Read the model definition and answer for the solid it produces. Units are mm, in the model's axes. A direction names the side the tool comes from. Coordinates: 2 decimals unless noted, no trailing zeros. Order: outer loops, then holes, each group sorted by start corner. A loop starts at its lowest first (then second) coordinate and runs counter-clockwise, first axis right, second up. Notation, with made-up numbers: M 78,72.25 L 97,72.25 A30 cw 97,100.25 Z; hole C -6,-14 d2. An arc over 180 degrees is marked long. Write each question's results on one line, items separated by ' | '.
```python
from build123d import *

# Parameters (mm, degrees)
F0_W     = 300
F0_H     = 15
F1_DEPTH = 10
F2_W     = 20
F2_H     = 15
F3_DEPTH = 10
F4_R     = 2.5
F5_DEPTH = 25
F6_R     = 2.5
F7_DEPTH = 25


with BuildPart() as f1:
    # F0 (on Front) → F1 (new body)
    with BuildSketch(Plane.XZ):
        Rectangle(F0_W, F0_H)
    extrude(amount=F1_DEPTH)

    # F2 (on face) → F3 (join)
    with BuildSketch(Plane(origin=(0, 0, 0), x_dir=(-1, 0, 0), z_dir=(0, 1, 0))):
        with Locations((-140, 0)):
            Rectangle(F2_W, F2_H)
        with Locations((140, 0)):
            Rectangle(F2_W, F2_H)
    extrude(amount=F3_DEPTH)

    # F4 (on face) → F5 (cut)
    with BuildSketch(Plane.XY.offset(7.5)):
        with Locations((140, 0)):
            Circle(F4_R)
        with Locations((-140, 0)):
            Circle(F4_R)
    extrude(amount=-F5_DEPTH, mode=Mode.SUBTRACT)

    # F6 (on face) → F7 (cut)
    with BuildSketch(Plane(origin=(0, 0, 0), x_dir=(-1, 0, 0), z_dir=(0, 1, 0))):
        with Locations((-25.5, 0)):
            Circle(F6_R)
        with Locations((25.5, 0)):
            Circle(F6_R)
    extrude(amount=-F7_DEPTH, mode=Mode.SUBTRACT)


solid = f1.part
```
(1) The part is cut by section D-D, the plane x = -124. Write down the section's boundary in (y, z).
Conclusion:
outline: M -10,-7.5 L 0,-7.5 L 0,7.5 L -10,7.5 Z
(2) Straight lines are drawn through the part: line 1 (X direction, y = 8.5, z = 5.5); line 2 (Y direction, x = 140, z = 4.75); line 3 (X direction, y = 1.5, z = 3.75). For each, find the intervals that lie inside material, in ascending order.
Conclusion:
line 1: -150 to -130, 130 to 150 | line 2: -10 to -2.5, 2.5 to 10 | line 3: -150 to -142, -138 to -130, 130 to 138, 142 to 150
(3) Given pin 1 (3 mm diameter, centred on x = 140, y = 0, fed in from -Z); pin 2 (7.5 mm diameter, centred on x = 15.5, z = -1, fed in from +Y), each flat-ended and moving along its own axis, determine where each tip first touches the part or whether it passes through.
Conclusion:
pin 1: through | pin 2: y = 0
(4) The part is cut by section A-A, the plane z = 0. Write down the section's boundary in (x, y).
Conclusion:
outline: M -150,-10 L -28,-10 L -28,0 L -130,0 L -130,10 L -150,10 Z; M -23,-10 L 23,-10 L 23,0 L -23,0 Z; M 28,-10 L 150,-10 L 150,10 L 130,10 L 130,0 L 28,0 Z; hole C -140,0 d5; hole C 140,0 d5
(5) For faces 1 (the cylindrical face through (-137.615, 0.751, 0.105)), 2 (the flat face through (130, 5, 0)), determine the directions among +Z, -Z, +X, -X, +Y, -Y from which every point of the face is accessible in a straight line to the end or side of a thin tool.
Conclusion:
face 1: +Z, -Z | face 2: +Z, -Z, +Y
(6) The mould has two halves that part along Y. Classify faces 3 (the flat face through (-130, 5, 0)), 4 (the flat face through (-2, 0, 0)), 5 (the cylindrical face through (142.385, 0.751, 0.105)): pulls with the +Y half, pulls with the -Y half, needs draft (parallel to the pull), parting line crosses it, or undercut.
Conclusion:
face 3: needs draft | face 4: pulls with the +Y half | face 5: undercut
(7) The part is cut by section B-B, the plane x = -25.5. Write down the section's boundary in (y, z).
Conclusion:
outline: M -10,-7.5 L 0,-7.5 L 0,-2.5 L -10,-2.5 Z; M -10,2.5 L 0,2.5 L 0,7.5 L -10,7.5 Z
(8) The part is cut by section C-C, the plane x = 140. Write down the section's boundary in (y, z).
Conclusion:
outline: M -10,-7.5 L -2.5,-7.5 L -2.5,7.5 L -10,7.5 Z; M 2.5,-7.5 L 10,-7.5 L 10,7.5 L 2.5,7.5 Z
